Read the model definition and answer for the solid it produces. Units are mm, in the model's axes. A direction names the side the tool comes from. Coordinates: 2 decimals unless noted, no trailing zeros. Write each loop counter-clockwise with the first axis right and the second up, starting at its lowest first coordinate (ties: lowest second). Pieces come first, ordered by that corner, then holes.
1) Find the intervals of material crossed by line 1 (X direction, y = -2.7, z = 0); line 2 (Z direction, x = 30.5, y = -2.25); line 3 (Z direction, x = 36.5, y = -5), in increasing order.
2) Each of these flat-tipped pins is pushed along its axis until it touches: pin 1 Ø4 at (y, z) = (2, -4.5) entering from -X; pin 2 Ø23 at (x, z) = (29.44, -17) entering from +Y; pin 3 Ø4.5 at (x, z) = (0, 0) entering from +Y. Where does it stop, or does it pass through?
3) Which of the six approach directions +Z, -Z, +X, -X, +Y, -Y give full straight-line access (tool end or side, diameter ignored) to faces 5 (the face through (-2, 0, -1)), 6 (the face through (-48, 6, 12))?
4) The part is cut by section B-B (y = 4.25). Determine the outline of the cut face in (x, z).
5) The part is cut by section A-A (x = 0). Give the number of separate pieces and of enclosed holes in the cut face, then the cut area to 3 significant figures.
6) Determine the mould class of faces 1 (the face through (20.57, -3.97, 21.61)), 2 (the face through (5, 6, 4)), 3 (the face through (-9.76, 4.03, -2.17)), 4 (the face through (-52.716, 0.084, -11.706)) for opening direction Z: +Z half, -Z half, draft (parallel to the pull), parting line (faces both ways), or undercut.
from build123d import *

# Parameters (mm, degrees)
SKETCH1_R           = 54
BOSS_EXTRUDE1_DEPTH = 6
SKETCH2_R           = 49
SKETCH2_R_2         = 10
CUT_EXTRUDE1_DEPTH  = 8
CUT_EXTRUDE2_DEPTH  = 6
SKETCH4_R           = 2
CUT_EXTRUDE3_DEPTH  = 6
SKETCH6_R           = 10
CUT_EXTRUDE5_DEPTH  = 4
FILLET1_R           = 4


with BuildPart() as part:
    # Sketch1 → Boss-Extrude1 (new, symmetric)
    with BuildSketch(Plane(origin=(0, 0, 0), x_dir=(1, 0, 0), z_dir=(0, 1, 0))):
        with Locations(Location((0, 0, 0), (0, 0, 270))):
            Circle(SKETCH1_R)
    extrude(amount=BOSS_EXTRUDE1_DEPTH, both=True)

    # Sketch2 → Cut-Extrude1 (cut)
    with BuildSketch(Plane(origin=(0, 6, 0), x_dir=(1, 0, 0), z_dir=(0, 1, 0))):
        with Locations(Location((0, 0, 0), (0, 0, 270))):
            Circle(SKETCH2_R)
        with Locations(Location((0, 0, 0), (0, 0, 270))):
            Circle(SKETCH2_R_2, mode=Mode.SUBTRACT)
    extrude(amount=-CUT_EXTRUDE1_DEPTH, mode=Mode.SUBTRACT)

    # Sketch3 → Cut-Extrude2 (cut)
    with BuildSketch(Plane(origin=(0, 6, 0), x_dir=(1, 0, 0), z_dir=(0, 1, 0))):
        Polygon((6.92820323, 0), (3.464101615, 6), (-3.464101615, 6), (-6.92820323, 0), (-3.464101615, -6), (3.464101615, -6), align=None)
    extrude(amount=-CUT_EXTRUDE2_DEPTH, mode=Mode.SUBTRACT)

    # Sketch4 → Cut-Extrude3 (cut)
    with BuildSketch(Plane(origin=(0, 0, 0), x_dir=(1, 0, 0), z_dir=(0, 1, 0))):
        with Locations(Location((0, 0, 0), (0, 0, 270))):
            Circle(SKETCH4_R)
    extrude(amount=-CUT_EXTRUDE3_DEPTH, mode=Mode.SUBTRACT)

    # Sketch6 → Cut-Extrude5 (cut)
    with BuildSketch(Plane(origin=(0, -2, 0), x_dir=(1, 0, 0), z_dir=(0, 1, 0))):
        with Locations(Location((0, 34, 0), (0, 0, 270))):
            Circle(SKETCH6_R)
        with Locations(Location((29.444863729, 17, 0), (0, 0, 270))):
            Circle(SKETCH6_R)
        with Locations(Location((29.444863729, -17, 0), (0, 0, 270))):
            Circle(SKETCH6_R)
        with Locations(Location((0, -34, 0), (0, 0, 270))):
            Circle(SKETCH6_R)
        with Locations(Location((-29.444863729, -17, 0), (0, 0, 270))):
            Circle(SKETCH6_R)
        with Locations(Location((-29.444863729, 17, 0), (0, 0, 270))):
            Circle(SKETCH6_R)
    extrude(amount=-CUT_EXTRUDE5_DEPTH, mode=Mode.SUBTRACT)

    # Fillet1
    fillet1_edges = [part.edges().sort_by_distance(p)[0] for p in [
        (0, -2, -49),
        (0, -2, -10),
    ]]
    fillet(fillet1_edges, radius=FILLET1_R)


solid = part.part
Reported:
1. line 1: x = -54 to -2, 2 to 54
1. line 2: z = -44.56 to -26.94, -7.06 to 7.06, 26.94 to 44.56
1. line 3: z = -39.8 to -24.09, -9.91 to 9.91, 24.09 to 39.8
2. pin 1: stops at x = -53.94
2. pin 2: stops at y = -1.97
2. pin 3: stops at y = 0
3. face 5: +Y
3. face 6: +Z, -Z, +X, -X, +Y
4. outline: circle Ø108 at (0, 0); circle Ø20 at (0, 0); hole circle Ø98 at (0, 0); hole (-6.93, 0) - (-3.46, -6) - (3.46, -6) - (6.93, 0) - (3.46, 6) - (-3.46, 6) - close
5. separate pieces: 4
5. enclosed holes: 0
5. area: 430 mm2
6. face 1: undercut
6. face 2: draft
6. face 3: undercut
6. face 4: parting line
